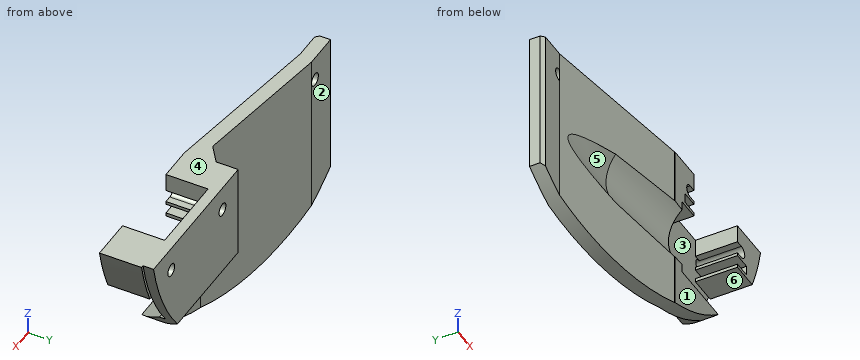
from build123d import *

# Parameters (mm, degrees)
SKETCH1_W            = 10
SKETCH1_H            = 10
BOSS_EXTRUDE1_DEPTH  = 4
CHAMFER1_SIZE        = 1
BOSS_EXTRUDE2_DEPTH  = 16
BOSS_EXTRUDE3_DEPTH  = 10
BOSS_EXTRUDE4_DEPTH  = 13
CHAMFER2_SIZE        = 10.3
BOSS_EXTRUDE5_DEPTH  = 30
CUT_EXTRUDE2_REACH   = 128.642
CUT_EXTRUDE1_START   = -15
CUT_EXTRUDE1_DEPTH   = 15
M3_CLEARANCE_HOLE1_D = 3.6
SKETCH11_W           = 1.8
SKETCH11_H           = 7.9
CHAMFER3_SIZE        = 5
CHAMFER3_SIZE2       = 4.40344093
BOSS_EXTRUDE6_DEPTH  = 12


# Read off the part's stored shape, not the designer's step: Cut-Extrude1
with BuildPart() as part:
    # Sketch1 → Boss-Extrude1 (new body)
    with BuildSketch(Plane(origin=(0, 0, 0), x_dir=(1, 0, 0), z_dir=(0, 1, 0))):
        with Locations((-5, 5)):
            Rectangle(SKETCH1_W, SKETCH1_H)
    extrude(amount=BOSS_EXTRUDE1_DEPTH)

    # Chamfer1
    chamfer1_edges = [part.edges().sort_by_distance(p)[0] for p in [
        (-10, 0, -5),
    ]]
    chamfer(chamfer1_edges, length=CHAMFER1_SIZE)

    # Sketch2 → Boss-Extrude2 (add)
    with BuildSketch(Plane(origin=(0, 0, -10), x_dir=(-1, 0, 0), z_dir=(0, 0, -1))):
        Polygon((10, 4), (0, 4), (-45.9, -2.784614526), (-45.9, 7.9), (-95.9, 7.9), (-95.9, 4.9), (-49.9, 4.9), (-49.9, -7.1), (-46.192330133, -7.1), (-46.146212438, -7.037883956), (1.467233005, 0), (9, 0), (10, 1), align=None)
    extrude(amount=BOSS_EXTRUDE2_DEPTH)

    # Sketch2<4> → Boss-Extrude3 (add)
    with BuildSketch(Plane(origin=(0, 0, -10), x_dir=(-1, 0, 0), z_dir=(0, 0, -1))):
        Polygon((1.467233005, 0), (0, 0), (0, 4), (-45.9, -2.784614526), (-45.9, 7.9), (-95.9, 7.9), (-95.9, 4.9), (-49.9, 4.9), (-49.9, -7.1), (-46.192330133, -7.1), (-46.146212438, -7.037883956), align=None)
    extrude(amount=-BOSS_EXTRUDE3_DEPTH)

    # Sketch3 → Boss-Extrude4 (add)
    with BuildSketch(Plane(origin=(0, 0, -26), x_dir=(-1, 0, 0), z_dir=(0, 0, -1))):
        Polygon((-95.9, 4.9), (-95.9, -7.1), (-49.9, -7.1), (-46.192330133, -7.1), (-46.146212438, -7.037883956), (1.467233005, 0), (9, 0), (10, 1), (10, 4), (0, 4), (-45.9, -2.784614526), (-45.9, 7.9), (-95.9, 7.9), align=None)
    extrude(amount=BOSS_EXTRUDE4_DEPTH)

    # Chamfer2
    chamfer2_edges = [part.edges().sort_by_distance(p)[0] for p in [
        (72.9, -7.1, -26),
    ]]
    chamfer(chamfer2_edges, length=CHAMFER2_SIZE)

    # Sketch4 → Boss-Extrude5 (add)
    with BuildSketch(Plane(origin=(0, 0, -39), x_dir=(-1, 0, 0), z_dir=(0, 0, -1))):
        Polygon((-95.9, 7.9), (-95.9, -7.1), (-46.192330133, -7.1), (-46.146212438, -7.037883956), (1.467233005, 0), (9, 0), (10, 1), (10, 4), (0, 4), (-45.9, -2.784614526), (-45.9, 7.9), align=None)
    extrude(amount=BOSS_EXTRUDE5_DEPTH)

    # Sketch15 → Cut-Extrude2 (cut, up to next)
    with BuildSketch(Plane(origin=(95.9, 0, 0), x_dir=(0, 0, -1), z_dir=(1, 0, 0)), mode=Mode.PRIVATE) as cut_extrude2_sk1:
        Polygon((69, -2.784614526), (37.641468776, -2.784614526), (26.956854249, 7.9), (69, 7.9), align=None)
    cut_extrude2_tool1 = extrude(cut_extrude2_sk1.sketch, amount=-CUT_EXTRUDE2_REACH, mode=Mode.PRIVATE) & part.part
    add(cut_extrude2_tool1.solids().sort_by_distance((95.9, 2.816908, -50.519973))[0], mode=Mode.SUBTRACT)

    # Cut-Extrude1 outline → Cut-Extrude1 (cut)
    with BuildSketch(Plane(origin=(0, 7.9, 0), x_dir=(1, 0, 0), z_dir=(0, 1, 0)).offset(CUT_EXTRUDE1_START)):
        with BuildLine():
            Line((90.528084846, 0), (95.9, 0))
            Line((95.9, 0), (95.9, 69))
            Line((95.9, 69), (-10, 69))
            Line((-10, 69), (-10, 41.287361933))
            ThreePointArc((-10, 41.287361933), (51.179168383, 47.220256879), (90.528084846, 0))
        make_face()
    extrude(amount=CUT_EXTRUDE1_DEPTH, mode=Mode.SUBTRACT)

    # M3 Clearance Hole1 (through all)
    with Locations(Plane(origin=(0, 4.9, 0), x_dir=(-1, 0, 0), z_dir=(0, -1, 0))):
        with Locations((-81.2, 7), (-54.2, 7)):
            Hole(M3_CLEARANCE_HOLE1_D / 2)

    # Sketch11 → M3 Clearance Hole2 (revolve, cut)
    with BuildSketch(Plane(origin=(-1.8, 0, -7), x_dir=(0, 0, -1), z_dir=(1, 0, 0))):
        with Locations((0.9, 3.95)):
            Rectangle(SKETCH11_W, SKETCH11_H)
    revolve(axis=Axis((-1.8, -6.35, -7), (0, 1, 0)), mode=Mode.SUBTRACT)

    # Chamfer3
    chamfer3_edges = [part.edges().sort_by_distance(p)[0] for p in [
        (45.9, -2.784614526, -18.820734388),
    ]]
    chamfer3_side = [part.faces().sort_by_distance(p)[0] for p in [
        (23.128110629, 0.581365679, -25.371340031),
    ]]
    chamfer(chamfer3_edges, length=CHAMFER3_SIZE, length2=CHAMFER3_SIZE2, reference=chamfer3_side[0])

    # Sketch12 → Cut-Revolve1 (revolve, cut)
    with BuildSketch(Plane.XY.offset(-25)):
        Polygon((0, -0.5), (22, -0.5), (92, -7.331568331), (90.828874, -19.331568331), (0, -10.467230343), align=None)
    revolve(axis=Axis((90.828874, -19.331568331, -25), (-0.9952714730097288, 0.09713235821828223, 0)), mode=Mode.SUBTRACT)

    # Sketch14 → Boss-Extrude6 (add)
    with BuildSketch(Plane.XZ.offset(-4.9)):
        with BuildLine():
            Line((49.9, 0), (49.9, -13.5))
            Line((49.9, -13.5), (56.25, -13.5))
            Line((56.25, -13.5), (56.25, -12.5))
            Line((56.25, -12.5), (51.45, -12.5))
            Line((51.45, -12.5), (51.45, -9.7))
            Line((51.45, -9.7), (56.25, -9.7))
            Line((56.25, -9.7), (56.25, -8.8))
            Line((56.25, -8.8), (54.2, -8.8))
            ThreePointArc((54.2, -8.8), (52.4, -7), (54.2, -5.2))
            Line((54.2, -5.2), (56.25, -5.2))
            Line((56.25, -5.2), (56.25, 0))
            Line((56.25, 0), (49.9, 0))
        make_face()
        with BuildLine():
            Line((79.15, -13.5), (86.943744534, -13.5))
            ThreePointArc((86.943744534, -13.5), (89.487636648, -6.866742476), (91.309542311, 0))
            Line((91.309542311, 0), (79.15, 0))
            Line((79.15, 0), (79.15, -5.2))
            Line((79.15, -5.2), (81.2, -5.2))
            ThreePointArc((81.2, -5.2), (83, -7), (81.2, -8.8))
            Line((81.2, -8.8), (79.15, -8.8))
            Line((79.15, -8.8), (79.15, -9.7))
            Line((79.15, -9.7), (83.95, -9.7))
            Line((83.95, -9.7), (83.95, -12.5))
            Line((83.95, -12.5), (79.15, -12.5))
            Line((79.15, -12.5), (79.15, -13.5))
        make_face()
    extrude(amount=BOSS_EXTRUDE6_DEPTH)


solid = part.part
Geometry: final body of the model. Coordinates: model frame, mm. Face numbers are marked on the shaded views. A direction names the side the tool comes from. Give positions to 0.01 mm unless a question says otherwise; leave off trailing zeros. Write each loop counter-clockwise with the first axis right and the second up, starting at its lowest first coordinate (ties: lowest second). Pieces come first, ordered by that corner, then holes.
(1) Cut plane A-A, the plane z = -45. Return loops of the section in (x, y), then the cut area to 3 significant figures.
(2) Cut plane B-B, the plane y = -5. Give the number of separate pieces and of enclosed holes in the cut face, then the cut area to 3 significant figures.
(3) Ray query, line 1 (Z direction, x = 81.2, y = 3); line 2 (Z direction, x = 54.2, y = -3.75); line 3 (Z direction, x = 54.2, y = 2). Return the intervals inside material, ascending.
(4) Mould query, pull axis Z, two halves, no side actions, for the marked faces 3, 4, 5 and 6. Classes: released by +Z, released by -Z, zero draft, split by the parting line, or undercut.
(5) First-contact query: P1, Ø1.5, axis at y = 5.5, z = -12.5, coming from the +X side; P2, Ø2.5, axis at x = 55, y = -4, coming from the -Z side; P3, Ø2, axis at x = 27.5, z = -44.5, coming from the +Y side. Flat tips, straight axial feed; report the tip coordinate or a pass-through.
(6) Access query for the marked faces 1 and 2. Directions: +Z, -Z, +X, -X, +Y, -Y. A direction counts if a zero-diameter tool reaches every point of the face in a straight line with its end or side. Return the directions, or none.
(7) Cut plane C-C, the plane z = -11. Return loops of the section in (x, y), then the cut area to 3 significant figures.
Values follow:
1. outline: (-3.62, 0) - (-1.47, 0) - (46.15, -7.04) - (46.19, -7.1) - (56.02, -7.1) - (56.02, -2.78) - (45.9, -2.78) - (0, 4) - (-3.62, 4) - close
1. area: 252 mm2
2. separate pieces: 3
2. enclosed holes: 0
2. area: 957 mm2
3. line 1: z = -13.5 to -12.5, -9.7 to -8.8, -5.2 to 0
3. line 2: z = -45.89 to -32.95, -13.5 to -12.5, -9.7 to -8.8, -5.2 to 0
3. line 3: z = -32.86 to -27.2, -13.5 to -12.5, -9.7 to -8.8, -5.2 to 0
4. face 3: undercut
4. face 4: released by +Z
4. face 5: undercut
4. face 6: released by -Z
5. P1: stops at x = 87.57
5. P2: stops at z = -46.1
5. P3: stops at y = 0.08
6. face 1: +Z, -Z, +X, -X, -Y
6. face 2: +Z, -Z, -X, +Y
7. outline: (-10, 1) - (-9, 0) - (-1.47, 0) - (46.15, -7.04) - (46.19, -7.1) - (51.45, -7.1) - (51.45, 4.9) - (83.95, 4.9) - (83.95, -7.1) - (88, -7.1) - (88, 4.9) - (87.17, 4.9) - (87.17, 7.9) - (45.9, 7.9) - (45.9, 1.62) - (40.95, -2.05) - (0, 4) - (-10, 4) - close
7. area: 483 mm2
